Here's how the part is built. I have some questions about the finished solid (model axes, mm). A direction names the side the tool comes from. Give positions to 0.01 mm unless a question says otherwise; leave off trailing zeros. Write each loop counter-clockwise with the first axis right and the second up, starting at its lowest first coordinate (ties: lowest second). Pieces come first, ordered by that corner, then holes. Notation, with made-up numbers: (-16.75, 31) - (25.25, 31) arc R30 cw to (25.25, 66) - close; hole circle Ø10 at (81, 28). An arc over 180 degrees is marked (long way). One line per item, written item: value. Start each with the question number.
1) Please list where these lines run through material, in increasing order: L1, parallel to X at y = 145, z = 15.5; L2, parallel to Z at x = 14.5, y = 12; L3, parallel to X at y = 39.5, z = 17. Write a range as [from, to].
2) I'm going to push flat-ended pins straight in: P1, Ø12, axis at x = 103.5, z = 26, coming from the -Y side; P2, Ø17.5, axis at x = 7, z = 18, coming from the +Y side; P3, Ø22.5, axis at y = 140.07, z = 67.14, coming from the -X side; P4, Ø12.5, axis at y = 31.79, z = -19.14, coming from the -X side. Where does each tip first touch, or does it pass through?
3) Imagine slicing it at C-C on z = -16.5. Write out the boundary of the cut face in (x, y), plus the area to 3 significant figures.
4) We'd pull the mould along Z, two halves only. Please class faces 1 (the flat face through (186, 87, 88)), 2 (the cylindrical face through (185.916, 16.944, -34.297)), 3 (the cylindrical face through (185.92, 32.1, 60.15)): +Z half, -Z half, draft (parallel to the pull), parting line (faces both ways), or undercut.
5) Imagine slicing it at B-B on x = 14.5. Write out the boundary of the cut face in (y, z), plus the area to 3 significant figures.
6) On a 3-axis mill with a long thin cutter (end or side, diameter ignored), from which of +Z, -Z, +X, -X, +Y, -Y can I reach the whole of each face in a straight line? I mean faces 4 (the flat face through (4, 25, 24)), 5 (the flat face through (114.052, 40.913, 3.987)). Say none if no direction works.
7) Imagine slicing it at D-D on y = 53.5. Write out the boundary of the cut face in (x, z), plus the area to 3 significant figures.
8) Imagine slicing it at A-A on y = 15. Write out the boundary of the cut face in (x, z).
from build123d import *

# Parameters (mm, degrees)
BOSS_EXTRUDE1_DEPTH      = 48
BOSS_EXTRUDE4_DEPTH      = 40
BOSS_EXTRUDE4_DEPTH_BACK = 88
FILLET2_R                = 20
SKETCH10_R               = 7
CUT_EXTRUDE3_DEPTH       = 40
CUT_EXTRUDE4_DEPTH       = 180
SKETCH12_R               = 10
CUT_EXTRUDE5_DEPTH       = 180


with BuildPart() as part:
    # Sketch1 → Boss-Extrude1 (new body)
    with BuildSketch(Plane.XY):
        with BuildLine():
            Line((0, 0), (0, 25.00039893))
            Line((0, 25.00039893), (22, 25.00039893))
            ThreePointArc((22, 25.00039893), (119.156102476, 50.883868102), (180, 130.929369905))
            Line((180, 130.929369905), (180, 56.026453851))
            ThreePointArc((180, 56.026453851), (105.819692691, 14.421228989), (22, 0))
            Line((22, 0), (0, 0))
        make_face()
    extrude(amount=BOSS_EXTRUDE1_DEPTH)

    # Sketch9 → Boss-Extrude4 (add, two sides: drawn at the far end of the back side and taken through both)
    with BuildSketch(Plane.XY.offset(48).offset(-BOSS_EXTRUDE4_DEPTH_BACK)):
        Polygon((180, 130.929369905), (180, 160.929369905), (192, 160.929369905), (192, 10.929369905), (180, 10.929369905), (180, 51.308831421), align=None)
    extrude(amount=BOSS_EXTRUDE4_DEPTH + BOSS_EXTRUDE4_DEPTH_BACK)

    # Fillet2
    fillet2_edges = [part.edges().sort_by_distance(p)[0] for p in [
        (186, 160.929369905, -40),
        (186, 10.929369905, -40),
        (186, 10.929369905, 88),
        (186, 160.929369905, 88),
    ]]
    fillet(fillet2_edges, radius=FILLET2_R)

    # Sketch10 → Cut-Extrude3 (cut)
    with BuildSketch(Plane.ZY.offset(-180)):
        with Locations((-19.142135624, 140.071505529)):
            Circle(SKETCH10_R)
        with Locations((67.142135624, 140.071505529)):
            Circle(SKETCH10_R)
        with Locations((67.142135624, 31.787234281)):
            Circle(SKETCH10_R)
        with Locations((-19.142135624, 31.787234281)):
            Circle(SKETCH10_R)
    extrude(amount=-CUT_EXTRUDE3_DEPTH, mode=Mode.SUBTRACT)

    # Sketch11 → Cut-Extrude4 (cut)
    with BuildSketch(Plane(origin=(0, 0, 0), x_dir=(1, 0, 0), z_dir=(0, 1, 0))):
        with BuildLine():
            ThreePointArc((9.39659903, -10.313017355), (2.718722307, -13.440381836), (0, -20.294796118))
            Line((0, -20.294796118), (0, 0))
            Line((0, 0), (180, 0))
            Line((180, 0), (9.39659903, -10.313017355))
        make_face()
        with BuildLine():
            ThreePointArc((9.39659903, -37.686982645), (2.718722307, -34.559618164), (0, -27.705203882))
            Line((0, -27.705203882), (0, -48))
            Line((0, -48), (180, -48))
            Line((180, -48), (9.39659903, -37.686982645))
        make_face()
    extrude(amount=CUT_EXTRUDE4_DEPTH, mode=Mode.SUBTRACT)

    # Sketch12 → Cut-Extrude5 (cut)
    with BuildSketch(Plane(origin=(0, 25.00039893, 0), x_dir=(1, 0, 0), z_dir=(0, 1, 0))):
        with Locations(Location((14.5, -24, 0), (0, 0, 41.409622109))):
            Circle(SKETCH12_R)
    extrude(amount=-CUT_EXTRUDE5_DEPTH, mode=Mode.SUBTRACT)


solid = part.part
Numbers:
1. L1: [180, 192]
1. L2: [10, 14], [34, 38]
1. L3: [99.09, 157.1], [180, 192]
2. P1: y = 11.63
2. P2: y = 25
2. P3: x = 180
2. P4: through
3. outline: (180, 10.93) - (192, 10.93) - (192, 25.31) - (180, 25.31) - close; (180, 38.27) - (192, 38.27) - (192, 133.59) - (180, 133.59) - close; (180, 146.55) - (192, 146.55) - (192, 160.93) - (180, 160.93) - close
3. area: 1,490 mm^2
4. face 1: +Z half
4. face 2: -Z half
4. face 3: undercut
5. outline: (0, 10) - (25, 10) - (25, 14) - (0, 14) - close; (0, 34) - (25, 34) - (25, 38) - (0, 38) - close
5. area: 200 mm^2
6. face 4: +Z, -Z, -X, +Y
6. face 5: -Z, -X, +Y, -Y
7. outline: (122.94, 3.45) - (176.83, 0.19) - (176.83, 47.81) - (122.94, 44.55) - close; (180, -40) - (192, -40) - (192, 88) - (180, 88) - close
7. area: 3,930 mm^2
8. outline: (0, 20.29) arc R10 ccw to (9.4, 10.31) - (107.43, 4.39) - (107.43, 43.61) - (9.4, 37.69) arc R10 ccw to (0, 27.71) - close; (180, -32.09) - (192, -32.09) - (192, 80.09) - (180, 80.09) - close; hole circle Ø20 at (14.5, 24)
